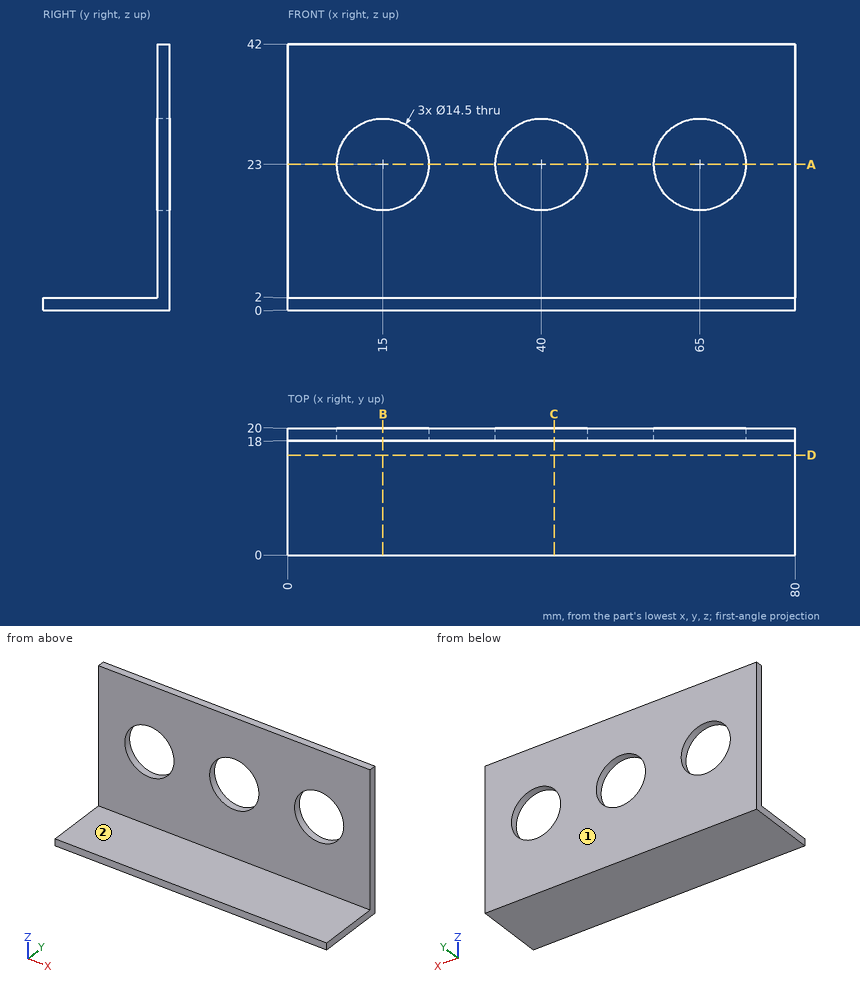
Geometry check sheet. Reference: drawing and pictorial views, mm from the part's lowest x, y, z. A direction names the side the tool comes from. Give positions to 0.01 mm unless a question says otherwise; leave off trailing zeros. Loops run counter-clockwise (first coordinate to the right, second up) from the corner with the lowest first, then second, coordinate; pieces in that order, holes last. Notation, with made-up numbers: (-29.75, 85.25) - (11.25, 85.25) arc R20 ccw to (11.25, 109.25) - close; hole circle Ø7 at (12, 62). An arc over 180 degrees is marked (long way). One line per question, with ' | ' between items. Start each with the question number.
1. Cross-section at A-A, the plane z = 23. Enter the section's corners in (x, y).
2. Gauge pin test, flat ends, axial feed: pin 1 Ø13 at (x, z) = (40, 23) entering from +Y; pin 2 Ø4 at (x, z) = (51, 36) entering from -Y; pin 3 Ø2 at (x, y) = (70.5, 16.5) entering from +Z. Record the tip position at first contact, or that the pin passes through.
3. Cross-section at B-B, the plane x = 15. Enter the section's corners in (y, z).
4. Set-up check for the marked faces 1 and 2: record each of +Z, -Z, +X, -X, +Y, -Y from which the full face is reachable in a straight line by a thin tool's end or side.
5. Material ranges on line 1 along X through (y, z) = (18.6, 23); line 2 along Z through (x, y) = (65, 19.65); line 3 along Y through (x, z) = (33.5, 13), recorded low to high. Write a range as [from, to].
6. Cross-section at D-D, the plane y = 15.75. Enter the section's corners in (x, z), plus the area to 3 significant figures.
7. Cross-section at C-C, the plane x = 42. Enter the section's corners in (y, z), plus the area to 3 significant figures.
Check result:
1) outline: (0, 18) - (7.75, 18) - (7.75, 20) - (0, 20) - close; (22.25, 18) - (32.75, 18) - (32.75, 20) - (22.25, 20) - close; (47.25, 18) - (57.75, 18) - (57.75, 20) - (47.25, 20) - close; (72.25, 18) - (80, 18) - (80, 20) - (72.25, 20) - close
2) pin 1: passes through | pin 2: stops at y = 18 | pin 3: stops at z = 2
3) outline: (0, 0) - (20, 0) - (20, 15.75) - (18, 15.75) - (18, 2) - (0, 2) - close; (18, 30.25) - (20, 30.25) - (20, 42) - (18, 42) - close
4) face 1: +Z, -Z, +X, -X, +Y | face 2: +Z, +X, -X, -Y
5) line 1: x = [0, 7.75], [22.25, 32.75], [47.25, 57.75], [72.25, 80] | line 2: z = [0, 15.75], [30.25, 42] | line 3: y = [18, 20]
6) outline: (0, 0) - (80, 0) - (80, 2) - (0, 2) - close | area: 160 mm2
7) outline: (0, 0) - (20, 0) - (20, 16.03) - (18, 16.03) - (18, 2) - (0, 2) - close; (18, 29.97) - (20, 29.97) - (20, 42) - (18, 42) - close | area: 92.1 mm2
